For this review, take the finished solid that the model builds, in its own axes (mm). A direction names the side the tool comes from. Coordinates: 2 decimals unless noted, no trailing zeros. Loops run counter-clockwise (first coordinate to the right, second up) from the corner with the lowest first, then second, coordinate; pieces in that order, holes last. Notation, with made-up numbers: M -0.75,29.5 L 8.25,29.5 A25 cw 8.25,68.5 Z; hole C 64,65 d1. An arc over 180 degrees is marked long. Write item = value, one per line.
from build123d import *

# Parameters (mm, degrees)
F0_R     = 11.0109
F0_R_2   = 4.0005284671
F1_DEPTH = 3.5052
F2_R     = 15.7206731231
F3_DEPTH = 4.43
F4_R     = 5.3773289571
F5_DEPTH = 25.4


with BuildPart() as f1:
    # F0 (on Front) → F1 (new body, symmetric)
    with BuildSketch(Plane.XZ):
        Circle(F0_R)
        Circle(F0_R_2, mode=Mode.SUBTRACT)
    extrude(amount=F1_DEPTH, both=True)

    # F2 (on Front) → F3 (join)
    with BuildSketch(Plane.XZ):
        Circle(F2_R)
    extrude(amount=F3_DEPTH)

    # F4 (on Front) → F5 (join)
    with BuildSketch(Plane.XZ):
        Circle(F4_R)
    extrude(amount=F5_DEPTH)


solid = f1.part
Q1. Add section C-C (y = -7.75). Write out the cut boundary in (x, z).
Solved:
outline = C 0,0 d10.75
Q2. Machinability: for faces 4 (the face through (5.919, 1.728, 9.284)), 5 (the face through (0, -25.4, 0)), 6 (the face through (0, -4.43, -7)), which of the approach directions +Z, -Z, +X, -X, +Y, -Y give a long, thin tool a straight path to every point of the face, cutting with its end or side? Answer none if there is none.
Solved:
face_4 = +Y
face_5 = +Z, -Z, +X, -X, -Y
face_6 = -Y
Q3. For line 1 along Z through (x, y) = (0, 1.95); line 2 along Y through (x, z) = (0, 8); line 3 along Y through (x, z) = (-12, -0.5), list the stretches that pass through material, from the lowest coordinate up.
Solved:
line_1 = -11.01 to -4, 4 to 11.01
line_2 = -4.43 to 3.51
line_3 = -4.43 to 0
Q4. Add section B-B (x = 0). Write out the cut boundary in (y, z).
Solved:
outline = M -25.4,-5.38 L -4.43,-5.38 L -4.43,-15.72 L 0,-15.72 L 0,-11.01 L 3.51,-11.01 L 3.51,-4 L 0,-4 L 0,4 L 3.51,4 L 3.51,11.01 L 0,11.01 L 0,15.72 L -4.43,15.72 L -4.43,5.38 L -25.4,5.38 Z
Q5. Draft analysis for pull direction X (two halves, no side actions). For faces 1 (the face through (3, 0, 11)), 2 (the face through (5.129, -14.768, 1.615)), 3 (the face through (-0.9, 1.8, -3.9)), state which applies: +X half, -X half, draft (parallel to the pull), parting line (faces both ways), or undercut.
Solved:
face_1 = draft
face_2 = parting line
face_3 = undercut
Q6. Add section D-D (x = 8). Write out the cut boundary in (y, z).
Solved:
outline = M -4.43,-13.53 L 0,-13.53 L 0,-7.57 L 3.51,-7.57 L 3.51,7.57 L 0,7.57 L 0,13.53 L -4.43,13.53 Z
Q7. Add section A-A (z = 0). Write out the cut boundary in (x, y).
Solved:
outline = M -15.72,-4.43 L -5.38,-4.43 L -5.38,-25.4 L 5.38,-25.4 L 5.38,-4.43 L 15.72,-4.43 L 15.72,0 L 11.01,0 L 11.01,3.51 L 4,3.51 L 4,0 L -4,0 L -4,3.51 L -11.01,3.51 L -11.01,0 L -15.72,0 Z
Q8. For pin 1 Ø4 at (y, z) = (-10.5, -1) entering from -X; pin 2 Ø6.5 at (x, z) = (0, 0) entering from +Y; pin 3 Ø3 at (x, y) = (-2.5, -16.5) entering from +Z, all flat-tipped, find the tip position at first contact; note any pin that passes through.
Solved:
pin_1 = -5.38
pin_2 = 0
pin_3 = 5.28
